Can you work these out from the model? Positions are in its coordinate system, mm. Round coordinates to 2 decimals unless told otherwise and drop trailing zeros. Order: outer loops, then holes, each group sorted by start corner. A loop starts at its lowest first (then second) coordinate and runs counter-clockwise, first axis right, second up.
Q1. Will these pins go through, and if not, where does the flat tip stop? P1, Ø6, axis at x = -40, z = 572, coming from the +Y side; P2, Ø4, axis at x = -44.5, y = -1.5, coming from the +Z side; P3, Ø3, axis at y = 5, z = 891, coming from the -X side.
Q2. If I drill on line 1 (Z direction, x = -51.75, y = 2.5); line 2 (Z direction, x = -42, y = -5.5); line 3 (Y direction, x = -45, z = 1177.5), over which ranges is the centre line in solid material (lowest first)?
Q3. If we section it at C-C (z = 666): Please give me the cut outline in (x, y), plus the area to 3 significant figures.
from build123d import *

# Parameters (mm, degrees)
BOSS_EXTRUDE1_START = 10
SKETCH1_R           = 8
BOSS_EXTRUDE1_DEPTH = 1200
CHAMFER1_SIZE       = 1
SKETCH2_R           = 4.25
CUT_EXTRUDE1_DEPTH  = 50
CUT_EXTRUDE2_START  = -50
SKETCH3_R           = 4.25
CUT_EXTRUDE2_DEPTH  = 50
CUT_EXTRUDE3_START  = -458.5
SKETCH4_R           = 8
SKETCH4_R_2         = 6
CUT_EXTRUDE3_DEPTH  = 15
CUT_EXTRUDE4_START  = -345
SKETCH4_2_R         = 8
SKETCH4_2_R_2       = 6
CUT_EXTRUDE4_DEPTH  = 15


with BuildPart() as part:
    # Sketch1 → Boss-Extrude1 (new body)
    with BuildSketch(Plane.XY.offset(BOSS_EXTRUDE1_START)):
        with Locations((-45, 0)):
            Circle(SKETCH1_R)
    extrude(amount=BOSS_EXTRUDE1_DEPTH)

    # Chamfer1
    chamfer1_edges = [part.edges().sort_by_distance(p)[0] for p in [
        (-53, 0, 10),
        (-53, 0, 1210),
    ]]
    chamfer(chamfer1_edges, length=CHAMFER1_SIZE)

    # Sketch2 → Cut-Extrude1 (cut)
    with BuildSketch(Plane.XY.offset(1210)):
        with Locations((-45, 0)):
            Circle(SKETCH2_R)
    extrude(amount=-CUT_EXTRUDE1_DEPTH, mode=Mode.SUBTRACT)

    # Sketch3 → Cut-Extrude2 (cut)
    with BuildSketch(Plane(origin=(0, 0, 10), x_dir=(-1, 0, 0), z_dir=(0, 0, -1)).offset(CUT_EXTRUDE2_START)):
        with Locations(Location((45, 0, 0), (0, 0, 180))):
            Circle(SKETCH3_R)
    extrude(amount=CUT_EXTRUDE2_DEPTH, mode=Mode.SUBTRACT)

    # Sketch4 → Cut-Extrude3 (cut)
    with BuildSketch(Plane.XY.offset(1210).offset(CUT_EXTRUDE3_START)):
        with Locations((-45, 0)):
            Circle(SKETCH4_R)
        with Locations((-45, 0)):
            Circle(SKETCH4_R_2, mode=Mode.SUBTRACT)
    extrude(amount=CUT_EXTRUDE3_DEPTH, mode=Mode.SUBTRACT)

    # Sketch4_2 → Cut-Extrude4 (cut)
    with BuildSketch(Plane.XY.offset(1210).offset(CUT_EXTRUDE4_START)):
        with Locations((-45, 0)):
            Circle(SKETCH4_2_R)
        with Locations((-45, 0)):
            Circle(SKETCH4_2_R_2, mode=Mode.SUBTRACT)
    extrude(amount=CUT_EXTRUDE4_DEPTH, mode=Mode.SUBTRACT)


solid = part.part
Solution:
1. P1: stops at y = 7.75
1. P2: stops at z = 1160
1. P3: stops at x = -52.19
2. line 1: z = 10.2 to 751.5, 766.5 to 865, 880 to 1209.8
2. line 2: z = 10 to 751.5, 766.5 to 865, 880 to 1210
2. line 3: y = -8 to -4.25, 4.25 to 8
3. outline: circle Ø16 at (-45, 0)
3. area: 201 mm2
